from build123d import *

# Parameters (mm, degrees)
SKETCH1_W                            = 50.8
SKETCH1_H                            = 21.844
STOCK_DEPTH                          = 23.749
CLEARANCE_HOLES_FOR_MOUNTING_BOLTS_D = 6.7564
SKETCH5_W                            = 50.8
SKETCH5_H                            = 4.7625
CLEARANCE_RABBIT_DEPTH               = 4.7625
SKETCH6_W                            = 11.3665
SKETCH6_H                            = 17.78
NUT_SLOT_DEPTH                       = 58.130946824


with BuildPart() as part:
    # Sketch1 → Stock (new body)
    with BuildSketch(Plane(origin=(0, 0, 0), x_dir=(1, 0, 0), z_dir=(0, 1, 0))):
        Rectangle(SKETCH1_W, SKETCH1_H)
    extrude(amount=STOCK_DEPTH)

    # Clearance holes for Mounting Bolts (through all)
    with Locations(Plane(origin=(0, 23.749, 0), x_dir=(1, 0, 0), z_dir=(0, 1, 0))):
        with Locations((-19.05, 0), (19.05, 0)):
            Hole(CLEARANCE_HOLES_FOR_MOUNTING_BOLTS_D / 2)

    # Sketch5 → Clearance Rabbit (cut)
    with BuildSketch(Plane.XZ):
        with Locations((0, 8.54075)):
            Rectangle(SKETCH5_W, SKETCH5_H)
        with Locations((0, -8.54075)):
            Rectangle(SKETCH5_W, SKETCH5_H)
    extrude(amount=-CLEARANCE_RABBIT_DEPTH, mode=Mode.SUBTRACT)

    # Sketch6 → Nut Slot (cut, through all)
    with BuildSketch(Plane(origin=(25.4, 0, 0), x_dir=(0, 0, -1), z_dir=(1, 0, 0))):
        with Locations((0, 23.749)):
            Rectangle(SKETCH6_W, SKETCH6_H)
    extrude(amount=-NUT_SLOT_DEPTH, mode=Mode.SUBTRACT)


solid = part.part
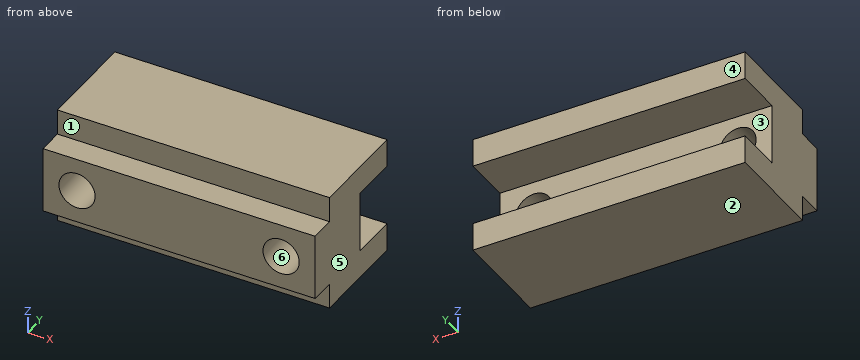
Here's how the part is built. I have some questions about the finished solid (model axes, mm). Face numbers are marked on the shaded views. A direction names the side the tool comes from. Coordinates: 2 decimals unless noted, no trailing zeros. Write each loop counter-clockwise with the first axis right and the second up, starting at its lowest first coordinate (ties: lowest second). Pieces come first, ordered by that corner, then holes.
Item 1: If I drill on line 1 (Z direction, x = -19.05, y = 8.5); line 2 (Z direction, x = 7.5, y = 18.5); line 3 (X direction, y = 11.25, z = -1), over which ranges is the centre line in solid material (lowest first)?
Item 2: I want a section at A-A on x = 19.05. Write out the boundary of the cut face in (y, z).
Item 3: I want a section at C-C on y = 19. Write out the boundary of the cut face in (x, z), and give its area (3 significant figures).
Item 4: On a 3-axis mill with a long thin cutter (end or side, diameter ignored), from which of +Z, -Z, +X, -X, +Y, -Y can I reach the whole of each face in a straight line? I mean the marked faces 1, 2 and 3. Say none if no direction works.
Item 5: Will these pins go through, and if not, where does the flat tip stop? pin 1 (1.4 mm diameter, centred on x = 2.5, z = -9, fed in from -Y); pin 2 (2.5 mm diameter, centred on x = -9, y = 3, fed in from -Z); pin 3 (11 mm diameter, centred on x = 19.05, z = 0, fed in from +Y).
Item 6: If we mould it in two halves opening along X, with no side actions, what happens to the marked faces 4, 5 and 6? For each: +X half, -X half, draft (parallel to the pull), parting line (faces both ways), or undercut.
Item 7: I want a section at D-D on y = 10.5. Write out the boundary of the cut face in (x, z).
Item 8: I want a section at B-B on z = 0. Write out the boundary of the cut face in (x, y).
Findings below:
1. line 1: z = -10.92 to -3.38, 3.38 to 10.92
1. line 2: z = -10.92 to -5.68, 5.68 to 10.92
1. line 3: x = -25.4 to -22.28, -15.82 to 15.82, 22.28 to 25.4
2. outline: (0, -6.16) - (4.76, -6.16) - (4.76, -10.92) - (23.75, -10.92) - (23.75, -5.68) - (14.86, -5.68) - (14.86, -3.38) - (0, -3.38) - close; (0, 3.38) - (14.86, 3.38) - (14.86, 5.68) - (23.75, 5.68) - (23.75, 10.92) - (4.76, 10.92) - (4.76, 6.16) - (0, 6.16) - close
3. outline: (-25.4, -10.92) - (25.4, -10.92) - (25.4, -5.68) - (-25.4, -5.68) - close; (-25.4, 5.68) - (25.4, 5.68) - (25.4, 10.92) - (-25.4, 10.92) - close
3. area: 532 mm2
4. face 1: +Z, +X, -X, -Y
4. face 2: -Z, +X, -X, +Y, -Y
4. face 3: +X, -X, +Y
5. pin 1: stops at y = 4.76
5. pin 2: stops at z = -6.16
5. pin 3: stops at y = 14.86
6. face 4: draft
6. face 5: +X half
6. face 6: undercut
7. outline: (-25.4, -10.92) - (25.4, -10.92) - (25.4, 10.92) - (-25.4, 10.92) - close; hole circle Ø6.76 at (-19.05, 0); hole circle Ø6.76 at (19.05, 0)
8. outline: (-25.4, 0) - (-22.43, 0) - (-22.43, 14.86) - (-25.4, 14.86) - close; (-15.67, 0) - (15.67, 0) - (15.67, 14.86) - (-15.67, 14.86) - close; (22.43, 0) - (25.4, 0) - (25.4, 14.86) - (22.43, 14.86) - close
